Build history of the part. All positions in model axes, mm. A direction names the side the tool comes from. Give positions to 0.01 mm unless a question says otherwise; leave off trailing zeros. Loops run counter-clockwise (first coordinate to the right, second up) from the corner with the lowest first, then second, coordinate; pieces in that order, holes last. Notation, with made-up numbers: (6.5, 0) - (22.5, 0) arc R8 cw to (22.5, 13) - close; hole circle Ø10 at (80, 37). An arc over 180 degrees is marked (long way). Return JSON: item names as keys, results as strings. Group by question number.
1) Slice it at C-C (x = 18.5). List the corners of the cut face in (y, z), and give its area (3 significant figures).
2) Slice it at B-B (z = -6). List the corners of the cut face in (x, y), and give its area (3 significant figures).
3) Slice it at A-A (y = -1). List the corners of the cut face in (x, z), and give its area (3 significant figures).
4) Drill centre lines: probe 1 along X at (y, z) = (18.75, 0) (3 decimals); probe 2 along X at (y, z) = (15.1, 15.5); probe 3 along Z at (x, y) = (-15.5, 13.65). Where is each one in solid material? Low to high. Write a range as from..to.
5) Mould opens along Y. For faces 4 (the face through (20.15, 0, 0)), 5 (the face through (-15, 12.5, 15)), 6 (the face through (-21.15, -12, 0)), 7 (the face through (0, -17, 0)) say: released by +Y, released by -Y, zero draft, split by the parting line, or undercut.
6) Drop flat-ended pins along their axis: pin 1 (1.1 mm diameter, centred on x = 2, z = -20.5, fed in from +Y); pin 2 (5 mm diameter, centred on x = 4, y = 33, fed in from -Z); pin 3 (1.1 mm diameter, centred on y = -13.5, z = -20.5, fed in from +X). Give the stop position or say it passes through.
7) Slice it at D-D (y = 10). List the corners of the cut face in (x, z), and give its area (3 significant figures).
8) 3-axis set-ups, long thin cutter, end or side, ignore diameter. For faces 1 (the face through (-15, 12.5, -16)), 2 (the face through (0, 0, -20.15)), 3 (the face through (-20.6, -7, 11)): which of +Z, -Z, +X, -X, +Y, -Y reach the whole face in a straight line?
```python
from build123d import *

# Parameters (mm, degrees)
EXTRUSION1_DEPTH      = 17
EXTRUSION1_DEPTH_BACK = 17
SKETCH2_R             = 11
EXTRUSION3_DEPTH      = 2
SKETCH3_R             = 4
EXTRUSION4_DEPTH      = 1
SKETCH4_R             = 3.175
EXTRUSION5_DEPTH      = 23
SKETCH5_W             = 30
SKETCH5_H             = 10
EXTRUSION6_DEPTH      = 1
SKETCH6_W             = 30
SKETCH6_H             = 10
EXTRUSION7_DEPTH      = 1
SKETCH7_W             = 7.283199846
SKETCH7_H             = 10
EXTRUSION8_DEPTH      = 1
EXTRUSION9_START      = -17
EXTRUSION9_DEPTH      = 10
EXTRUSION9_START_2    = 7
EXTRUSION9_2_DEPTH    = 10
EXTRUSION10_START     = -17
EXTRUSION10_DEPTH     = 10
EXTRUSION10_START_2   = 7
EXTRUSION10_2_DEPTH   = 10
HOLE3_D               = 3
HOLE3_DEPTH           = 4.5
EXTRUSION12_START     = -15
EXTRUSION12_DEPTH     = 15


# Read off the part's stored shape, not the designer's step: Extrusion9, Extrusion10
with BuildPart() as part:
    # Sketch1 → Extrusion1 (new, two sides: drawn at the far end of the back side and taken through both)
    with BuildSketch(Plane(origin=(0, 0, 0), x_dir=(-1, 0, 0), z_dir=(0, 1, 0)).offset(-EXTRUSION1_DEPTH_BACK)):
        Polygon((15, 20.15), (20.15, 15), (20.15, -15), (15, -20.15), (-15, -20.15), (-20.15, -15), (-20.15, 15), (-15, 20.15), align=None)
    extrude(amount=EXTRUSION1_DEPTH + EXTRUSION1_DEPTH_BACK)

    # Sketch2 → Extrusion3 (add)
    with BuildSketch(Plane(origin=(0, 17, 0), x_dir=(-1, 0, 0), z_dir=(0, 1, 0))):
        with Locations(Location((0, 0, 0), (0, 0, 90))):
            Circle(SKETCH2_R)
    extrude(amount=EXTRUSION3_DEPTH)

    # Sketch3 → Extrusion4 (cut)
    with BuildSketch(Plane(origin=(0, 19, 0), x_dir=(-1, 0, 0), z_dir=(0, 1, 0))):
        with Locations(Location((0, 0, 0), (0, 0, 90))):
            Circle(SKETCH3_R)
    extrude(amount=-EXTRUSION4_DEPTH, mode=Mode.SUBTRACT)

    # Sketch4 → Extrusion5 (add)
    with BuildSketch(Plane(origin=(0, 18, 0), x_dir=(-1, 0, 0), z_dir=(0, 1, 0))):
        with Locations(Location((0, 0, 0), (0, 0, 90))):
            Circle(SKETCH4_R)
    extrude(amount=EXTRUSION5_DEPTH)

    # Sketch5 → Extrusion6 (add)
    with BuildSketch(Plane.XY.offset(20.15)):
        with Locations((0, 12)):
            Rectangle(SKETCH5_W, SKETCH5_H)
        with Locations((0, -12)):
            Rectangle(SKETCH5_W, SKETCH5_H)
    extrusion6 = extrude(amount=EXTRUSION6_DEPTH)

    # Mirror1: Extrusion6 across plane
    add(extrusion6.mirror(Plane.XY))

    # Sketch6 → Extrusion7 (add)
    with BuildSketch(Plane(origin=(20.15, 0, 0), x_dir=(0, 0, -1), z_dir=(1, 0, 0))):
        with Locations((0, 12)):
            Rectangle(SKETCH6_W, SKETCH6_H)
        with Locations((0, -12)):
            Rectangle(SKETCH6_W, SKETCH6_H)
    extrusion7 = extrude(amount=EXTRUSION7_DEPTH)

    # Mirror2: Extrusion7 across plane
    add(extrusion7.mirror(Plane(origin=(0, 0, 0), x_dir=(0, 0, 1), z_dir=(1, 0, 0))))

    # Sketch7 → Extrusion8 (add)
    with BuildSketch(Plane(origin=(-17.575, 0, 17.575), x_dir=(0.7071067811865475, 0, 0.7071067811865477), z_dir=(-0.7071067811865477, 0, 0.7071067811865475))):
        with Locations((0, 12)):
            Rectangle(SKETCH7_W, SKETCH7_H)
        with Locations((0, -12)):
            Rectangle(SKETCH7_W, SKETCH7_H)
    extrude(amount=EXTRUSION8_DEPTH)

    # Extrusion9 outline → Extrusion9 (add)
    with BuildSketch(Plane(origin=(0, 0, 0), x_dir=(1, 0, 0), z_dir=(0, 1, 0)).offset(EXTRUSION9_START)):
        Polygon((-15.414213562, -21.15), (-15, -21.15), (-15, -20.15), (-15.707106781, -20.857106781), align=None)
    extrude(amount=EXTRUSION9_DEPTH)

    # Extrusion9 2 outline → Extrusion9 2 (add)
    with BuildSketch(Plane(origin=(0, 0, 0), x_dir=(1, 0, 0), z_dir=(0, 1, 0)).offset(EXTRUSION9_START_2)):
        Polygon((-15.414213562, -21.15), (-15, -21.15), (-15, -20.15), (-15.707106781, -20.857106781), align=None)
    extrude(amount=EXTRUSION9_2_DEPTH)

    # Extrusion10 outline → Extrusion10 (add)
    with BuildSketch(Plane(origin=(0, 0, 0), x_dir=(1, 0, 0), z_dir=(0, 1, 0)).offset(EXTRUSION10_START)):
        Polygon((-20.15, -15), (-21.15, -15), (-21.15, -15.414213562), (-20.857106781, -15.707106781), align=None)
    extrude(amount=EXTRUSION10_DEPTH)

    # Extrusion10 2 outline → Extrusion10 2 (add)
    with BuildSketch(Plane(origin=(0, 0, 0), x_dir=(1, 0, 0), z_dir=(0, 1, 0)).offset(EXTRUSION10_START_2)):
        Polygon((-20.15, -15), (-21.15, -15), (-21.15, -15.414213562), (-20.857106781, -15.707106781), align=None)
    extrude(amount=EXTRUSION10_2_DEPTH)

    # Hole3
    with Locations(Plane(origin=(0, 17, 0), x_dir=(1, 0, 0), z_dir=(0, 1, 0))):
        with Locations((-15.5, -15.5), (-15.5, 15.5), (15.5, 15.5), (15.5, -15.5)):
            Hole(HOLE3_D / 2, depth=HOLE3_DEPTH)

    # Sketch12 → Extrusion12 (cut)
    with BuildSketch(Plane(origin=(0, 41, 0), x_dir=(-1, 0, 0), z_dir=(0, 1, 0)).offset(EXTRUSION12_START)):
        with BuildLine():
            Line((-2.885307609, 1.325), (2.885307609, 1.325))
            ThreePointArc((2.885307609, 1.325), (0, 3.175), (-2.885307609, 1.325))
        make_face()
    extrude(amount=EXTRUSION12_DEPTH, mode=Mode.SUBTRACT)


solid = part.part
```
Results:
{
 "1": {"outline": "(-17, -16.65) - (17, -16.65) - (17, 16.65) - (-17, 16.65) - close", "area": "1,130 mm2"},
 "2": {"outline": "(-21.15, -17) - (21.15, -17) - (21.15, -7) - (20.15, -7) - (20.15, 7) - (21.15, 7) - (21.15, 17) - (9.22, 17) - (9.22, 19) - (-9.22, 19) - (-9.22, 17) - (-21.15, 17) - (-21.15, 7) - (-20.15, 7) - (-20.15, -7) - (-21.15, -7) - close", "area": "1,450 mm2"},
 "3": {"outline": "(-20.15, -15) - (-15, -20.15) - (15, -20.15) - (20.15, -15) - (20.15, 15) - (15, 20.15) - (-15, 20.15) - (-20.15, 15) - close", "area": "1,570 mm2"},
 "4": {"probe 1": "-11..-4, -3.175..3.175, 4..11", "probe 2": "-21.06..-17, -14..14, 17..19.65", "probe 3": "-19.65..-17, -14..14, 17..21.06"},
 "5": {"face 4": "undercut", "face 5": "released by +Y", "face 6": "zero draft", "face 7": "released by -Y"},
 "6": {"pin 1": "y = 17", "pin 2": "z = -2.8", "pin 3": "x = 15.2"},
 "7": {"outline": "(-21.15, -15) - (-20.15, -15) - (-15, -20.15) - (-15, -21.15) - (15, -21.15) - (15, -20.15) - (20.15, -15) - (21.15, -15) - (21.15, 15) - (20.15, 15) - (15, 20.15) - (15, 21.15) - (-15.41, 21.15) - (-21.15, 15.41) - close", "area": "1,700 mm2"},
 "8": {"face 1": "+Y", "face 2": "-Z, +X, -X", "face 3": "+Z, -X"}
}
